Read the model definition and answer for the solid it produces. Units are mm, in the model's axes. A direction names the side the tool comes from. Give positions to 0.01 mm unless a question says otherwise; leave off trailing zeros. Write each loop counter-clockwise with the first axis right and the second up, starting at its lowest first coordinate (ties: lowest second). Pieces come first, ordered by that corner, then holes. Notation, with made-up numbers: M -23.5,-26.5 L -12.5,-26.5 A22 cw -12.5,-8.5 Z; hole C -27,-19.75 d1. An arc over 180 degrees is marked long. Use a Markdown table: item, result. Add a question column.
Item 1: A cutting plane is placed at C-C on y = -57.5. Determine the outline of the cut face in (x, z) (1 decimal).
Item 2: Given P1, Ø8, axis at x = -1, z = -3.5, coming from the +Y side; P2, Ø4, axis at x = -4.5, y = -76, coming from the -Z side; P3, Ø4, axis at y = -18.5, z = 5, coming from the +X side, each flat-ended and moving along its own axis, determine where each tip first touches the part or whether it passes through.
Item 3: Consider probe 1 along Y at (x, z) = (-1, 7.75) (3 decimals); probe 2 along X at (y, z) = (-48.5, -6.25); probe 3 along Z at (x, y) = (-0.5, -114). Determine where each line is inside the solid, lowest interval first. Write a range as [from, to].
Item 4: For faces 1 (the flat face through (0, -111.125, 7)), 2 (the cylindrical face through (-1.72, -69.29, -7.75)), 3 (the flat face through (0, -28.6, 7)), determine the directions among +Z, -Z, +X, -X, +Y, -Y from which every point of the face is accessible in a straight line to the end or side of a thin tool.
from build123d import *

# Parameters (mm, degrees)
F0_R     = 7.9375
F1_DEPTH = 136.525
F2_R     = 7.9375
F2_R_2   = 6.35
F3_DEPTH = 25.4
F4_R     = 7.9375
F4_R_2   = 6.35
F5_DEPTH = 28.6004


with BuildPart() as f1:
    # F0 (on Front) → F1 (new body)
    with BuildSketch(Plane.XZ):
        Circle(F0_R)
    extrude(amount=F1_DEPTH)

    # F2 (on face) → F3 (cut)
    with BuildSketch(Plane.XZ.offset(136.525)):
        Circle(F2_R)
        Circle(F2_R_2, mode=Mode.SUBTRACT)
    extrude(amount=-F3_DEPTH, mode=Mode.SUBTRACT)

    # F4 (on face) → F5 (cut)
    with BuildSketch(Plane(origin=(0, 0, 0), x_dir=(-1, 0, 0), z_dir=(0, 1, 0))):
        Circle(F4_R)
        Circle(F4_R_2, mode=Mode.SUBTRACT)
    extrude(amount=-F5_DEPTH, mode=Mode.SUBTRACT)


solid = f1.part
Filled in:
| question | item | result |
|---|---|---|
| 1 | outline | C 0,0 d15.9 |
| 2 | P1 | y = 0 |
| 2 | P2 | z = -7.53 |
| 2 | P3 | x = 5.6 |
| 3 | probe 1 | [-111.125, -28.6] |
| 3 | probe 2 | [-4.89, 4.89] |
| 3 | probe 3 | [-6.33, 6.33] |
| 4 | face 1 | -Y |
| 4 | face 2 | +Y, -Y |
| 4 | face 3 | +Y |
